Part print with two shaded views. Sizes in mm from the minimum x, y, z corner. A direction names the side the tool comes from. Coordinates: 2 decimals unless noted, no trailing zeros. Loops run counter-clockwise (first coordinate to the right, second up) from the corner with the lowest first, then second, coordinate; pieces in that order, holes last. Notation, with made-up numbers: (-10.75, 22) -> (8.25, 22) arc R8 ccw to (8.25, 33) -> close; hole circle Ø1 at (62.5, -13.5). An arc over 180 degrees is marked (long way). Use one line per item in the form item = value.
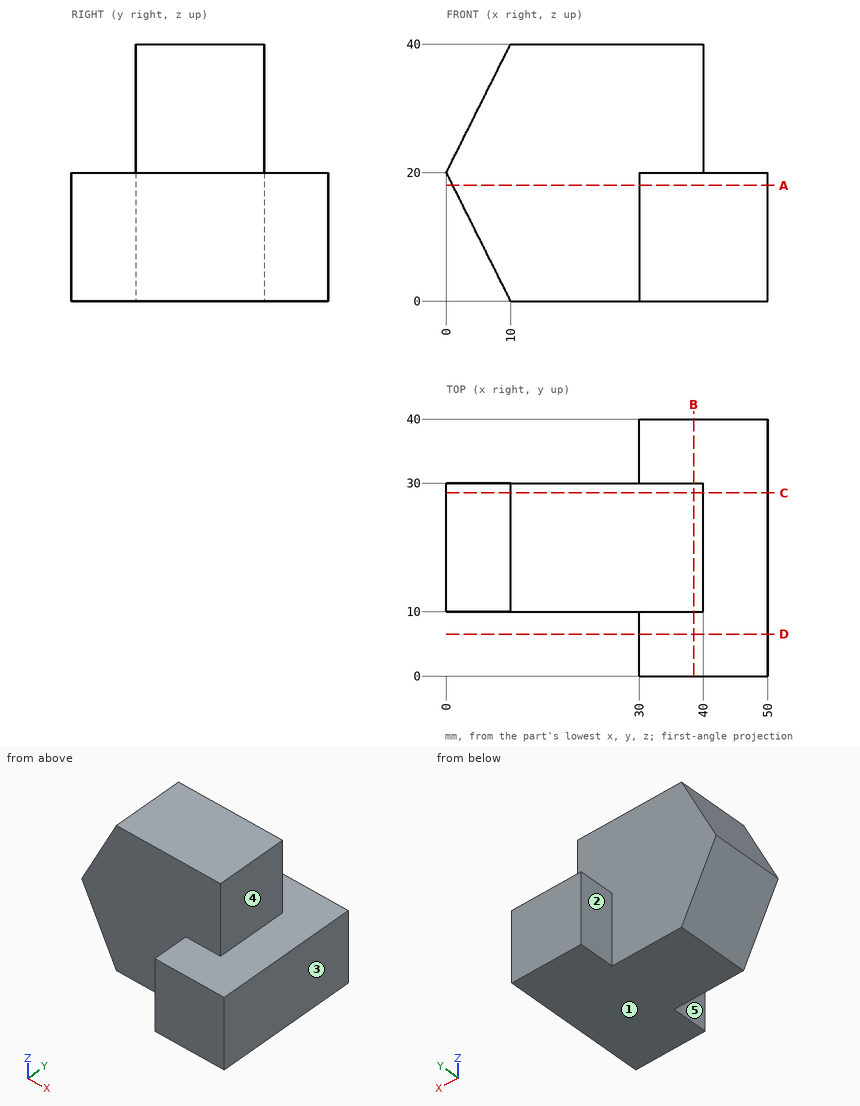
Q1. Pin check, flat tips, straight feed: pin 1 Ø6 at (x, y) = (44.5, 13) entering from +Z; pin 2 Ø1 at (x, z) = (10.5, 29.5) entering from -Y; pin 3 Ø3 at (y, z) = (18, 19) entering from -X; pin 4 Ø12 at (x, z) = (29.5, 17.5) entering from -Y. Stop position of each tip, or through.
Result:
pin_1 = 20
pin_2 = 10
pin_3 = 0
pin_4 = 0
Q2. Band-saw the part on B-B, the plane x = 38.5. Write the cut outline in (y, z).
Result:
outline = (0, 0) -> (40, 0) -> (40, 20) -> (30, 20) -> (30, 40) -> (10, 40) -> (10, 20) -> (0, 20) -> close
Q3. Which spindle directions (+Z, -Z, +X, -X, +Y, -Y) get a long thin tool onto all of the face, cutting with end or side? Do the marked faces 1, 2, 3, 4 and 5. Say none if no direction does.
Result:
face_1 = -Z, +X, -X, +Y, -Y
face_2 = +Z, -Z, -X, +Y
face_3 = +Z, -Z, +X, +Y, -Y
face_4 = +Z, +X, +Y, -Y
face_5 = +Z, -Z, -X, -Y
Q4. Band-saw the part on C-C, the plane y = 28.5. Write the cut outline in (x, z), and give its area (3 significant figures).
Result:
outline = (0, 20) -> (10, 0) -> (50, 0) -> (50, 20) -> (40, 20) -> (40, 40) -> (10, 40) -> close
area = 1,600 mm2
Q5. Wall check: line 1 along Z through (x, y) = (47, 5.5); line 2 along Y through (x, z) = (26, 21); line 3 along X through (y, z) = (34.5, 12). Give the ranges that are in metal, low to high.
Result:
line_1 = 0 to 20
line_2 = 10 to 30
line_3 = 30 to 50
Q6. Band-saw the part on D-D, the plane y = 6.5. Write the cut outline in (x, z).
Result:
outline = (30, 0) -> (50, 0) -> (50, 20) -> (30, 20) -> close
Q7. Band-saw the part on A-A, the plane z = 18. Write the cut outline in (x, y).
Result:
outline = (1, 10) -> (30, 10) -> (30, 0) -> (50, 0) -> (50, 40) -> (30, 40) -> (30, 30) -> (1, 30) -> close
